Source: three-view drawing plus pictorial views. Frame: mm from the lowest corner of the part. Give positions to 0.01 mm unless a question says otherwise; leave off trailing zeros. Write each loop counter-clockwise with the first axis right and the second up, starting at its lowest first coordinate (ties: lowest second). Pieces come first, ordered by that corner, then holes.
Q1. Cut plane B-B on z = 44. Return the cut outline in (x, y).
Q2. Pin query (flat end, axial travel): pin 1 (10 mm diameter, centred on x = 230.5, z = 31, fed in from +Y). Return the tip coordinate at first contact, or that it passes through.
Q3. Cut plane A-A on y = 17. Return the cut outline in (x, z), plus the area to 3 significant figures.
Q4. Cut plane C-C on x = 215. Return the cut outline in (y, z), plus the area to 3 significant figures.
Q5. Line query: L1, parallel to Z at x = 148, y = 7; L2, parallel to X at y = 9, z = 112; L3, parallel to X at y = 13, z = 124. Output: solid intervals per line, ascending.
Q6. Draft query along Z for the marked faces 1, 2, 3 and 4. Return one class per face: pulls with the +Z half, pulls with the -Z half, needs draft (parallel to the pull), parting line crosses it, or undercut.
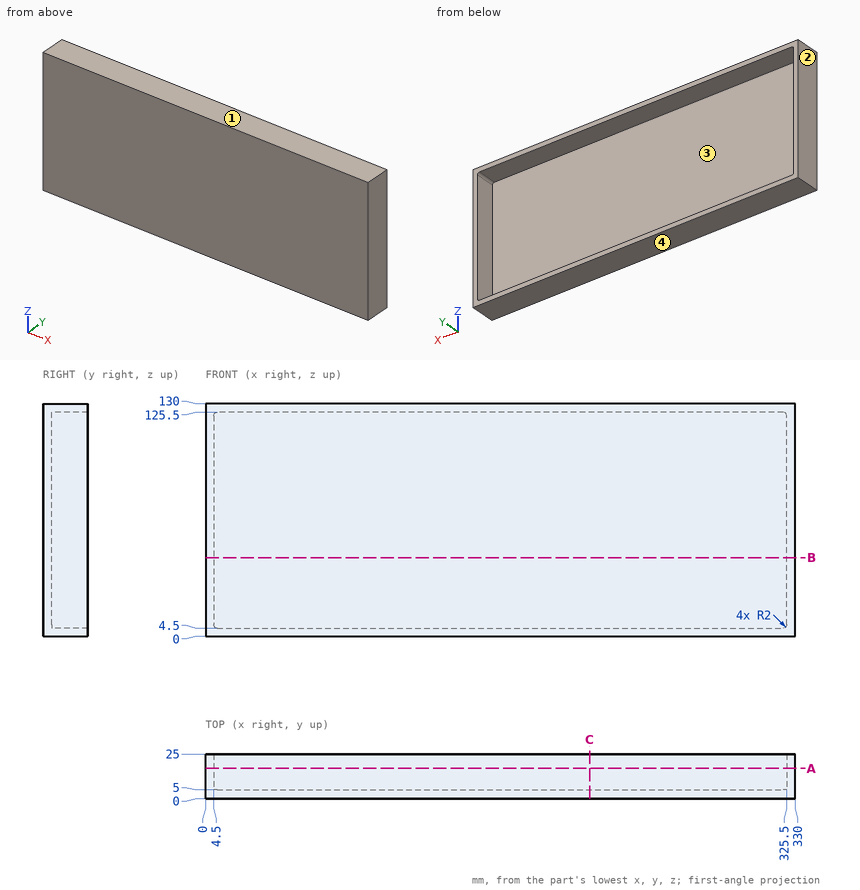
Data:
1. outline: (0, 0) - (330, 0) - (330, 25) - (325.5, 25) - (325.5, 5) - (4.5, 5) - (4.5, 25) - (0, 25) - close
2. pin 1: stops at y = 5
3. outline: (0, 0) - (330, 0) - (330, 130) - (0, 130) - close; hole (4.5, 6.5) arc R2 ccw to (6.5, 4.5) - (323.5, 4.5) arc R2 ccw to (325.5, 6.5) - (325.5, 123.5) arc R2 ccw to (323.5, 125.5) - (6.5, 125.5) arc R2 ccw to (4.5, 123.5) - close
3. area: 4,060 mm2
4. outline: (0, 0) - (25, 0) - (25, 4.5) - (5, 4.5) - (5, 125.5) - (25, 125.5) - (25, 130) - (0, 130) - close
4. area: 830 mm2
5. L1: z = 0 to 4.5, 125.5 to 130
5. L2: x = 0 to 4.5, 325.5 to 330
5. L3: x = 0 to 4.56, 325.44 to 330
6. face 1: pulls with the +Z half
6. face 2: needs draft
6. face 3: undercut
6. face 4: pulls with the -Z half
